```python
from build123d import *

# Parameters (mm, degrees)
F0_R     = 31.1006600455
F0_R_2   = 25.4231956913
F1_DEPTH = 7.6
F2_R     = 5
F3_R     = 0.5


with BuildPart() as f1:
    # F0 (on Front) → F1 (new body, symmetric)
    with BuildSketch(Plane.XZ):
        Circle(F0_R)
        Circle(F0_R_2, mode=Mode.SUBTRACT)
    extrude(amount=F1_DEPTH, both=True)

    # F2
    f2_edges = [f1.edges().sort_by_distance(p)[0] for p in [
        (-31.10066, 7.6, 0),
        (31.10066, 0, 0),
        (-31.10066, -7.6, 0),
    ]]
    fillet(f2_edges, radius=F2_R)

    # F3
    f3_edges = [f1.edges().sort_by_distance(p)[0] for p in [
        (-25.423196, -7.6, 0),
        (25.423196, 0, 0),
        (-25.423196, 7.6, 0),
    ]]
    fillet(f3_edges, radius=F3_R)


solid = f1.part
```
Here's how the part is built. I have some questions about the finished solid (model axes, mm). Give positions to 0.01 mm unless a question says otherwise; leave off trailing zeros. Write each loop counter-clockwise with the first axis right and the second up, starting at its lowest first coordinate (ties: lowest second). Pieces come first, ordered by that corner, then holes. Notation, with made-up numbers: (41, 36.5) -> (58, 36.5) arc R21 cw to (58, 71.5) -> close; hole circle Ø9 at (42.25, 35.25). An arc over 180 degrees is marked (long way). Use one line per item in the form item = value.
1) If I drill on L1, parallel to Z at x = 0, y = -2.5; L2, parallel to X at y = -2, z = 17.5; L3, parallel to Z at x = 3.5, y = 6.25, over which ranges is the centre line in solid material (lowest first)? Write a range as [from, to].
Verdict:
L1 = [-31.1, -25.42], [25.42, 31.1]
L2 = [-25.71, -18.44], [18.44, 25.71]
L3 = [-29.31, -25.18], [25.18, 29.31]
2) We'd pull the mould along Z, two halves only. Please class faces 1 (the face through (24.25, 0.1, 7.64)), 2 (the face through (-24.7, 0, -18.9)): +Z half, -Z half, draft (parallel to the pull), parting line (faces both ways), or undercut.
Verdict:
face_1 = undercut
face_2 = parting line
3) Suppose I cut it at A-A (z = 0). Please give me the cut outline in (x, y).
Verdict:
outline = (-31.1, -2.6) arc R5 ccw to (-26.1, -7.6) -> (-25.92, -7.6) arc R0.5 ccw to (-25.42, -7.1) -> (-25.42, 7.1) arc R0.5 ccw to (-25.92, 7.6) -> (-26.1, 7.6) arc R5 ccw to (-31.1, 2.6) -> close; (25.42, -7.1) arc R0.5 ccw to (25.92, -7.6) -> (26.1, -7.6) arc R5 ccw to (31.1, -2.6) -> (31.1, 2.6) arc R5 ccw to (26.1, 7.6) -> (25.92, 7.6) arc R0.5 ccw to (25.42, 7.1) -> close
4) Suppose I cut it at B-B (x = 0). Please give me the cut outline in (y, z), and give its area (3 significant figures).
Verdict:
outline = (-7.6, -26.1) arc R5 ccw to (-2.6, -31.1) -> (2.6, -31.1) arc R5 ccw to (7.6, -26.1) -> (7.6, -25.92) arc R0.5 ccw to (7.1, -25.42) -> (-7.1, -25.42) arc R0.5 ccw to (-7.6, -25.92) -> close; (-7.6, 25.92) arc R0.5 ccw to (-7.1, 25.42) -> (7.1, 25.42) arc R0.5 ccw to (7.6, 25.92) -> (7.6, 26.1) arc R5 ccw to (2.6, 31.1) -> (-2.6, 31.1) arc R5 ccw to (-7.6, 26.1) -> close
area = 151 mm2
5) Suppose I cut it at C-C (y = -1). Please give me the cut outline in (x, z).
Verdict:
outline = circle Ø62.2 at (0, 0); hole circle Ø50.85 at (0, 0)
6) I'm going to push flat-ended pins straight in: pin 1 (6 mm diameter, centred on x = 11, y = 4, fed in from +Z); pin 2 (3 mm diameter, centred on y = 5, z = -23.5, fed in from -X); pin 3 (5 mm diameter, centred on x = -15, y = 2, fed in from +Z). Where does each tip first touch, or does it pass through?
Verdict:
pin_1 = 29.99
pin_2 = -21.38
pin_3 = 28.48
